Check sheet for the modelled part. Datum: model origin and axes. Units: mm. Face numbers are marked on the shaded views. A direction names the side the tool comes from. Round coordinates to 2 decimals unless told otherwise and drop trailing zeros. Write each loop counter-clockwise with the first axis right and the second up, starting at its lowest first coordinate (ties: lowest second). Pieces come first, ordered by that corner, then holes.
Item 1: Section check B-B, the plane z = -82. Record the cut outline in (x, y) (3 decimals).
Item 2: Depth check by flat-ended pin: pin 1 (2.5 mm diameter, centred on x = 420, z = -30.93, fed in from -Y); pin 2 (2.5 mm diameter, centred on y = -8.235, z = -31.6, fed in from +X) (3 decimals). Enter the tip coordinate at first touch or a pass-through.
Item 3: Section check A-A, the plane y = -20. Record the cut outline in (x, z) (3 decimals), plus the area to 3 significant figures.
Item 4: Section check D-D, the plane x = 251.5. Record the cut outline in (y, z) (3 decimals).
Item 5: Set-up check for the marked faces 5 and 6: record each of +Z, -Z, +X, -X, +Y, -Y from which the full face is reachable in a straight line by a thin tool's end or side.
Item 6: Section check C-C, the plane x = 177. Record the cut outline in (y, z) (3 decimals), plus the area to 3 significant figures.
Item 7: Release check for a two-part mould opening along X. For the marked faces 1, 2, 3 and 4 record: pulls with the +X half, pulls with the -X half, needs draft (parallel to the pull), parting line crosses it, or undercut.
Item 8: Material ranges on line 1 along Z through (x, y) = (20, -0.9) (3 decimals); line 2 along Y through (x, z) = (381, -24) (3 decimals); line 3 along Y through (x, z) = (270, -134.5) (3 decimals), recorded low to high.
from build123d import *

# Parameters (mm, degrees)
F0_W      = 440
F0_H      = 88.87
F0_R      = 10
F0_R_2    = 1.6
F0_W_2    = 12
F0_H_2    = 4.5
F0_R_3    = 11
F1_DEPTH  = 0.635
F2_W      = 440
F2_H      = 152.87
F2_R      = 2.1
F3_DEPTH  = 0.635
F4_W      = 440
F4_H      = 152.87
F4_W_2    = 232.765
F4_H_2    = 112.87
F4_W_3    = 122.235
F4_H_3    = 122.87
F5_DEPTH  = 0.635
F6_W      = 440
F6_H      = 87.6
F7_DEPTH  = 0.635
F8_W      = 440
F8_H      = 30.965
F8_R      = 2.1
F9_DEPTH  = 0.635
F11_W     = 31.6
F11_H     = 121.27
F11_R     = 2.1
F12_DEPTH = 0.635
F13_DEPTH = 0.635
F14_W     = 12.1
F14_H     = 152.235
F14_R     = 1.5
F15_DEPTH = 0.635


with BuildPart() as f1:
    # F0 (on Top) → F1 (new body)
    with BuildSketch(Plane.XY):
        with Locations((220, -44.435)):
            Rectangle(F0_W, F0_H)
        with Locations((20, -20)):
            Circle(F0_R, mode=Mode.SUBTRACT)
        with Locations((190.92939, -12.25)):
            Circle(F0_R_2, mode=Mode.SUBTRACT)
        with Locations((205.92939, -12.25)):
            Rectangle(F0_W_2, F0_H_2, mode=Mode.SUBTRACT)
        with Locations((246.765, -44.435)):
            Circle(F0_R_3, mode=Mode.SUBTRACT)
        with Locations((220.92939, -12.25)):
            Circle(F0_R_2, mode=Mode.SUBTRACT)
    extrude(amount=F1_DEPTH)

    # F2 (on Front) → F3 (join)
    with BuildSketch(Plane.XZ):
        with Locations((220, -76.435)):
            Rectangle(F2_W, F2_H)
        with Locations((20, -132.87)):
            Circle(F2_R, mode=Mode.SUBTRACT)
        with Locations((265.143272, -132.87)):
            Circle(F2_R, mode=Mode.SUBTRACT)
        with Locations((20, -20)):
            Circle(F2_R, mode=Mode.SUBTRACT)
        with Locations((420, -30.92768)):
            Circle(F2_R, mode=Mode.SUBTRACT)
    extrude(amount=F3_DEPTH)

    # F4 (on face) → F5 (join)
    with BuildSketch(Plane.XZ.offset(88.87)):
        with Locations((220, -76.435)):
            Rectangle(F4_W, F4_H)
        with Locations((161.3825, -76.435)):
            Rectangle(F4_W_2, F4_H_2, mode=Mode.SUBTRACT)
        with Locations((368.8825, -86.435)):
            Rectangle(F4_W_3, F4_H_3, mode=Mode.SUBTRACT)
    extrude(amount=-F5_DEPTH)

    # F6 (on face) → F7 (join)
    with BuildSketch(Plane(origin=(0, 0, -152.87), x_dir=(1, 0, 0), z_dir=(0, 0, -1))):
        with Locations((220, 44.435)):
            Rectangle(F6_W, F6_H)
    extrude(amount=-F7_DEPTH)

    # F8 (on face) → F9 (join)
    with BuildSketch(Plane.XZ.offset(0.635)):
        with Locations((220, -136.7525)):
            Rectangle(F8_W, F8_H)
        with Locations((20, -132.87)):
            Circle(F8_R, mode=Mode.SUBTRACT)
        with Locations((265.143272, -132.87)):
            Circle(F8_R, mode=Mode.SUBTRACT)
    extrude(amount=F9_DEPTH)

    # F11 (on face) → F12 (join)
    with BuildSketch(Plane.XZ.offset(0.635)):
        with Locations((15.8, -60.635)):
            Rectangle(F11_W, F11_H)
        with Locations((20, -20)):
            Circle(F11_R, mode=Mode.SUBTRACT)
    extrude(amount=F12_DEPTH)

    # F10 (on face) → F13 (join)
    with BuildSketch(Plane(origin=(0, 0, 0), x_dir=(0, -1, 0), z_dir=(-1, 0, 0))):
        Polygon((88.235, 0), (0.635, 0), (0.635, -121.27), (1.27, -121.27), (1.27, -152.235), (88.235, -152.235), align=None)
    extrude(amount=-F13_DEPTH)

    # F14 (on face) → F15 (join)
    with BuildSketch(Plane.YZ.offset(440)):
        with Locations((-82.185, -76.1175)):
            Rectangle(F14_W, F14_H)
        with Locations((-80.635, -144.635)):
            Circle(F14_R, mode=Mode.SUBTRACT)
        with Locations((-80.635, -7.6)):
            Circle(F14_R, mode=Mode.SUBTRACT)
        Polygon((-0.635, 0), (-12.735, 0), (-12.735, -152.235), (-1.27, -152.235), (-1.27, -121.27), (-0.635, -121.27), align=None)
        with Locations((-8.235, -31.6)):
            Circle(F14_R, mode=Mode.SUBTRACT)
    extrude(amount=-F15_DEPTH)


solid = f1.part
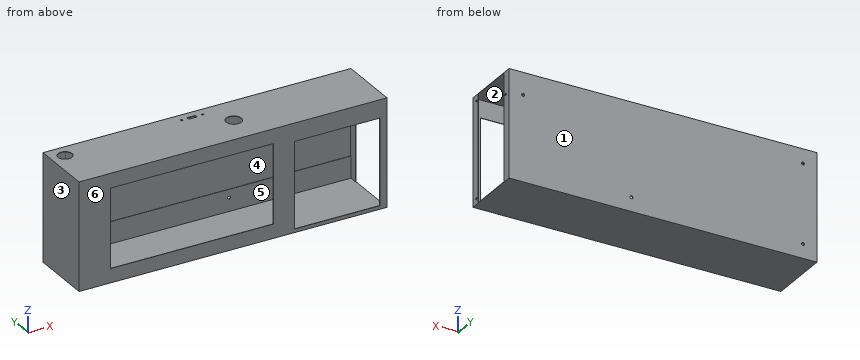
Values found:
1. outline: (0, -88.87) - (45, -88.87) - (45, -88.235) - (0.635, -88.235) - (0.635, -1.27) - (31.6, -1.27) - (31.6, -0.635) - (439.365, -0.635) - (439.365, -12.735) - (440, -12.735) - (440, 0) - (0, 0) - close; (277.765, -88.87) - (307.765, -88.87) - (307.765, -88.235) - (277.765, -88.235) - close; (430, -88.87) - (440, -88.87) - (440, -76.135) - (439.365, -76.135) - (439.365, -88.235) - (430, -88.235) - close
2. pin 1: passes through
2. pin 2: stops at x = 0.635
3. outline: (0, -152.87) - (440, -152.87) - (440, -152.235) - (0.635, -152.235) - (0.635, 0) - (10, 0) - (10, 0.635) - (0, 0.635) - close; (30, 0) - (440, 0) - (440, 0.635) - (30, 0.635) - close
3. area: 643 mm2
4. outline: (-88.87, -152.87) - (0, -152.87) - (0, 0.635) - (-34.506, 0.635) - (-34.506, 0) - (-0.635, 0) - (-0.635, -121.27) - (-1.27, -121.27) - (-1.27, -152.235) - (-88.235, -152.235) - (-88.235, -132.87) - (-88.87, -132.87) - close; (-88.87, -20) - (-88.235, -20) - (-88.235, 0) - (-54.364, 0) - (-54.364, 0.635) - (-88.87, 0.635) - close
5. face 5: none
5. face 6: +Z, -Z, +X, -X, -Y
6. outline: (-88.87, -152.87) - (0, -152.87) - (0, 0.635) - (-88.87, 0.635) - (-88.87, -20) - (-88.235, -20) - (-88.235, 0) - (-0.635, 0) - (-0.635, -121.27) - (-1.27, -121.27) - (-1.27, -152.235) - (-88.235, -152.235) - (-88.235, -132.87) - (-88.87, -132.87) - close
6. area: 254 mm2
7. face 1: needs draft
7. face 2: undercut
7. face 3: pulls with the -X half
7. face 4: undercut
8. line 1: z = -152.87 to -134.97, -130.77 to -22.1, -17.9 to 0.635
8. line 2: y = -88.87 to -88.235, -0.635 to 0
8. line 3: y = -88.87 to -88.235, -1.27 to 0
